For this review, take the finished solid that the model builds, in its own axes (mm). A direction names the side the tool comes from. Coordinates: 2 decimals unless noted, no trailing zeros. Write each loop counter-clockwise with the first axis right and the second up, starting at its lowest first coordinate (ties: lowest second). Pieces come first, ordered by that corner, then holes.
```python
from build123d import *

# Parameters (mm, degrees)
F0_R     = 1
F1_DEPTH = 4
F2_R     = 4
F3_DEPTH = 1


with BuildPart() as f1:
    # F0 (on Top) → F1 (new body)
    with BuildSketch(Plane.XY):
        Polygon((7.764571, 28.977775), (0, 20), (-7.764571, 28.977775), (-10, 17.320508), (-21.213203, 21.213203), (-17.320508, 10), (-28.977775, 7.764571), (-20, 0), (-28.977775, -7.764571), (-17.320508, -10), (-21.213203, -21.213203), (-10, -17.320508), (-7.764571, -28.977775), (0, -20), (7.764571, -28.977775), (10, -17.320508), (21.213203, -21.213203), (17.320508, -10), (28.977775, -7.764571), (20, 0), (28.977775, 7.764571), (17.320508, 10), (21.213203, 21.213203), (10, 17.320508), align=None)
        Circle(F0_R, mode=Mode.SUBTRACT)
    extrude(amount=F1_DEPTH)

    # F2 (on face) → F3 (cut)
    with BuildSketch(Plane.XY.offset(4)):
        Polygon((-13.34884, -7.706956), (-16.348923, -16.348923), (-7.706956, -13.34884), (-5.984121, -22.333044), (0, -15.413913), (5.984121, -22.333044), (7.706956, -13.34884), (16.348923, -16.348923), (13.34884, -7.706956), (22.333044, -5.984121), (15.413913, 0), (22.333044, 5.984121), (13.34884, 7.706956), (16.348923, 16.348923), (7.706956, 13.34884), (5.984121, 22.333044), (0, 15.413913), (-5.984121, 22.333044), (-7.706956, 13.34884), (-16.348923, 16.348923), (-13.34884, 7.706956), (-22.333044, 5.984121), (-15.413913, 0), (-22.333044, -5.984121), align=None)
        Circle(F2_R, mode=Mode.SUBTRACT)
    extrude(amount=-F3_DEPTH, mode=Mode.SUBTRACT)


solid = f1.part
```
Q1. Clearance check with flat-ended pins moving along their axes: pin 1 Ø1.5 at (x, z) = (13, 2) entering from -Y; pin 2 Ø1.6 at (x, y) = (0, 0) entering from +Z; pin 3 Ø1 at (x, z) = (5.5, 1.5) entering from -Y; pin 4 Ø1 at (y, z) = (15, 0.5) entering from +X. State where each tip first meets the part, or that it passes through.
Ans:
pin 1: stops at y = -18.62
pin 2: passes through
pin 3: stops at y = -26.94
pin 4: stops at x = 19.23
Q2. Add section A-A (y = -5). State the section outline as (x, z) points, then the cut area to 3 significant figures.
Ans:
outline: (-25.78, 0) - (25.78, 0) - (25.78, 4) - (21.2, 4) - (21.2, 3) - (-21.2, 3) - (-21.2, 4) - (-25.78, 4) - close
area: 164 mm2
Q3. For probe 1 along X at (y, z) = (3.5, 3.55); probe 2 along Y at (x, z) = (-0.5, 3.15); probe 3 along Z at (x, y) = (-3, 3.5), list the stretches that pass through material, from the lowest coordinate up.
Ans:
probe 1: x = -24.05 to -19.46, -1.94 to 1.94, 19.46 to 24.05
probe 2: y = -20.58 to -15.99, -3.97 to -0.87, 0.87 to 3.97, 15.99 to 20.58
probe 3: z = 0 to 3
Q4. Tool access review of faces 1 (the flat face through (17.778, -6.858, 3.507)), 2 (the flat face through (-3.83, 24.43, 1.97)), 3 (the flat face through (24.43, 3.83, 1.97)): name each direction out of +Z, -Z, +X, -X, +Y, -Y from which nothing blocks a thin tool from reaching the whole face with its end or side.
Ans:
face 1: +Z
face 2: +Z, -Z, +Y
face 3: +Z, -Z, +X
Q5. Draft analysis for pull direction X (two halves, no side actions). For faces 4 (the flat face through (19.24, 15.53, 1.97)), 5 (the flat face through (-14.87, 12.09, 3.51)), 6 (the flat face through (-23.231, -8.867, 1.972)), 7 (the flat face through (-9, 15, 4)), state which applies: +X half, -X half, draft (parallel to the pull), parting line (faces both ways), or undercut.
Ans:
face 4: +X half
face 5: undercut
face 6: -X half
face 7: draft
